Build history of the part. All positions in model axes, mm. A direction names the side the tool comes from. Coordinates: 2 decimals unless noted, no trailing zeros. Loops run counter-clockwise (first coordinate to the right, second up) from the corner with the lowest first, then second, coordinate; pieces in that order, holes last.
(1) Tool access for faces 4 (the face through (-4.769, -21.477, 1.183)), 5 (the face through (0, 0, -0.6)): list every direction of +Z, -Z, +X, -X, +Y, -Y with a clear straight run to the whole face (end or side of a thin tool).
(2) Flat gauge pins, fed straight in: P1, Ø1.5, axis at y = -7.5, z = -7.5, coming from the +X side; P2, Ø6, axis at y = 7.5, z = -10, coming from the -X side; P3, Ø8, axis at x = 13.5, z = -7, coming from the +Y side; P4, Ø5, axis at x = 0, y = 17.5, coming from the -Z side. Where does each tip first touch, or does it go through?
(3) Two-plate mould, pull along X, no slides. Class faces 1 (the face through (-2.38, -10.74, -8.42)), 2 (the face through (-10, -5, 0)), 3 (the face through (-0.358, 20.227, 1.217)): pulls with the +X half, pulls with the -X half, needs draft (parallel to the pull), parting line crosses it, or undercut.
(4) Slice it at C-C (y = -8.75). Give the cut face in (x, z), and give its area (3 significant figures).
(5) Slice it at B-B (y = 0). Give the cut face in (x, z).
(6) Wall check: L1, parallel to Y at x = 0, z = 1.1; L2, parallel to Z at x = -11.5, y = 3.5; L3, parallel to Y at x = 0, z = -9.5. Give the ranges that are in metal, low to high.
(7) Slice it at A-A (x = 0). Give the cut face in (y, z).
(8) Slice it at D-D (x = 7). Give the cut face in (y, z), and give its area (3 significant figures).
from build123d import *

# Parameters (mm, degrees)
SKETCH1_R           = 22
SKETCH1_R_2         = 11
BOSS_EXTRUDE1_DEPTH = 2.4
SKETCH2_R           = 2.75
CUT_EXTRUDE1_DEPTH  = 32.205127784
BOSS_EXTRUDE4_START = -19
SKETCH4_R           = 11
BOSS_EXTRUDE4_DEPTH = 19
SKETCH6_R           = 5.4
CUT_EXTRUDE2_DEPTH  = 3


with BuildPart() as part:
    # Sketch1 → Boss-Extrude1 (new body)
    with BuildSketch(Plane.XY):
        Circle(SKETCH1_R)
        Circle(SKETCH1_R_2, mode=Mode.SUBTRACT)
    extrude(amount=BOSS_EXTRUDE1_DEPTH)

    # Sketch2 → Cut-Extrude1 (cut, through all)
    with BuildSketch(Plane.XY.offset(2.4)):
        with Locations((0, 17.5)):
            Circle(SKETCH2_R)
        with Locations((15.155444566, -8.75)):
            Circle(SKETCH2_R)
        with Locations((-15.155444566, -8.75)):
            Circle(SKETCH2_R)
    extrude(amount=-CUT_EXTRUDE1_DEPTH, mode=Mode.SUBTRACT)

    # Sketch4 → Boss-Extrude4 (add)
    with BuildSketch(Plane.XY.offset(2.4).offset(BOSS_EXTRUDE4_START)):
        Circle(SKETCH4_R)
    extrude(amount=BOSS_EXTRUDE4_DEPTH)

    # Sketch6 → Cut-Extrude2 (cut)
    with BuildSketch(Plane.XY.offset(2.4)):
        Circle(SKETCH6_R)
    extrude(amount=-CUT_EXTRUDE2_DEPTH, mode=Mode.SUBTRACT)


solid = part.part
Response values:
1. face 4: +Z, -Z
1. face 5: +Z
2. P1: stops at x = 8.69
2. P2: stops at x = -10.04
2. P3: stops at y = 5.55
2. P4: passes through
3. face 1: parting line crosses it
3. face 2: needs draft
3. face 3: undercut
4. outline: (-20.19, 0) - (-17.91, 0) - (-17.91, 2.4) - (-20.19, 2.4) - close; (-12.41, 0) - (-6.67, 0) - (-6.67, -16.6) - (6.67, -16.6) - (6.67, 0) - (12.41, 0) - (12.41, 2.4) - (-12.41, 2.4) - close; (17.91, 0) - (20.19, 0) - (20.19, 2.4) - (17.91, 2.4) - close
4. area: 292 mm2
5. outline: (-22, 0) - (-11, 0) - (-11, -16.6) - (11, -16.6) - (11, 0) - (22, 0) - (22, 2.4) - (5.4, 2.4) - (5.4, -0.6) - (-5.4, -0.6) - (-5.4, 2.4) - (-22, 2.4) - close
6. L1: y = -22 to -5.4, 5.4 to 14.75, 20.25 to 22
6. L2: z = 0 to 2.4
6. L3: y = -11 to 11
7. outline: (-22, 0) - (-11, 0) - (-11, -16.6) - (11, -16.6) - (11, 0) - (14.75, 0) - (14.75, 2.4) - (5.4, 2.4) - (5.4, -0.6) - (-5.4, -0.6) - (-5.4, 2.4) - (-22, 2.4) - close; (20.25, 0) - (22, 0) - (22, 2.4) - (20.25, 2.4) - close
8. outline: (-20.86, 0) - (-8.49, 0) - (-8.49, -16.6) - (8.49, -16.6) - (8.49, 0) - (20.86, 0) - (20.86, 2.4) - (-20.86, 2.4) - close
8. area: 382 mm2
